Source: CAD feature listing. Evaluate the final solid. Frame: model axes, mm. Round coordinates to 2 decimals unless told otherwise and drop trailing zeros. Order: outer loops, then holes, each group sorted by start corner. A loop starts at its lowest first (then second) coordinate and runs counter-clockwise, first axis right, second up. Notation, with made-up numbers: (22.5, 77) - (60.5, 77) arc R14 ccw to (60.5, 99) - close; hole circle Ø10 at (22, -16.5). An arc over 180 degrees is marked (long way). Return JSON: item names as keys, results as strings. Group by question number.
1) Section D-D, the plane x = 53.5. Return loops of the section in (y, z), plus the area to 3 significant figures.
2) Section A-A, the plane z = -17.5. Return loops of the section in (x, y).
3) Ray query, line 1 (Z direction, x = 0, y = 0.65); line 2 (Z direction, x = -65, y = 1.4); line 3 (X direction, y = 1, z = 19.5). Return the intervals inside material, ascending. Write a range as from..to.
4) Section B-B, the plane x = -65. Return loops of the section in (y, z), plus the area to 3 significant figures.
5) Section C-C, the plane y = 0.9. Give the number of separate pieces and of enclosed holes in the cut face, plus the area to 3 significant figures.
6) Contact query for flat-ended pins moving along their axis: P1, Ø5.5, axis at x = 30.31, z = -17.5, coming from the -Y side; P2, Ø20, axis at x = -65, z = -38, coming from the +Y side; P3, Ø1, axis at x = -58, y = 1.5, coming from the +Z side. Output: stop coordinate, or through.
```python
from build123d import *

# Parameters (mm, degrees)
F1_R     = 6.25
F1_R_2   = 3
F2_DEPTH = 2


with BuildPart() as f2:
    # F1 (on Front) → F2 (new body)
    with BuildSketch(Plane.XZ):
        with BuildLine():
            Line((-60, 67.371839), (-70, 67.371839))
            ThreePointArc((-70, 67.371839), (-77.071068, 64.442907), (-80, 57.371839))
            Line((-80, 57.371839), (-80, 0))
            Line((-80, 0), (-80, -43))
            ThreePointArc((-80, -43), (-77.071068, -50.071068), (-70, -53))
            Line((-70, -53), (0, -53))
            Line((0, -53), (70, -53))
            ThreePointArc((70, -53), (77.071068, -50.071068), (80, -43))
            Line((80, -43), (80, 0))
            Line((80, 0), (80, 57.371839))
            ThreePointArc((80, 57.371839), (77.071068, 64.442907), (70, 67.371839))
            Line((70, 67.371839), (60, 67.371839))
            ThreePointArc((60, 67.371839), (52.928932, 64.442907), (50, 57.371839))
            Line((50, 57.371839), (50, 56.150236))
            ThreePointArc((50, 56.150236), (47.666959, 50.503505), (42.028607, 48.150288))
            Line((42.028607, 48.150288), (0, 48))
            Line((0, 48), (-42.028607, 48.150288))
            ThreePointArc((-42.028607, 48.150288), (-47.666959, 50.503505), (-50, 56.150236))
            Line((-50, 56.150236), (-50, 57.371839))
            ThreePointArc((-50, 57.371839), (-52.928932, 64.442907), (-60, 67.371839))
        make_face()
        with Locations((-65, -38)):
            Circle(F1_R, mode=Mode.SUBTRACT)
        with Locations((-30.310889, -17.5)):
            Circle(F1_R_2, mode=Mode.SUBTRACT)
        with Locations((0, -35)):
            Circle(F1_R_2, mode=Mode.SUBTRACT)
        with Locations((65, -38)):
            Circle(F1_R, mode=Mode.SUBTRACT)
        with Locations((30.310889, -17.5)):
            Circle(F1_R_2, mode=Mode.SUBTRACT)
        with Locations((-30.310889, 17.5)):
            Circle(F1_R_2, mode=Mode.SUBTRACT)
        with Locations((-65, 52.371839)):
            Circle(F1_R, mode=Mode.SUBTRACT)
        with Locations((30.310889, 17.5)):
            Circle(F1_R_2, mode=Mode.SUBTRACT)
        with BuildLine():
            ThreePointArc((3, 35), (-2.12132, 32.87868), (0, 38))
            ThreePointArc((0, 38), (2.12132, 37.12132), (3, 35))
        make_face(mode=Mode.SUBTRACT)
        with Locations((65, 52.371839)):
            Circle(F1_R, mode=Mode.SUBTRACT)
    extrude(amount=-F2_DEPTH)


solid = f2.part
```
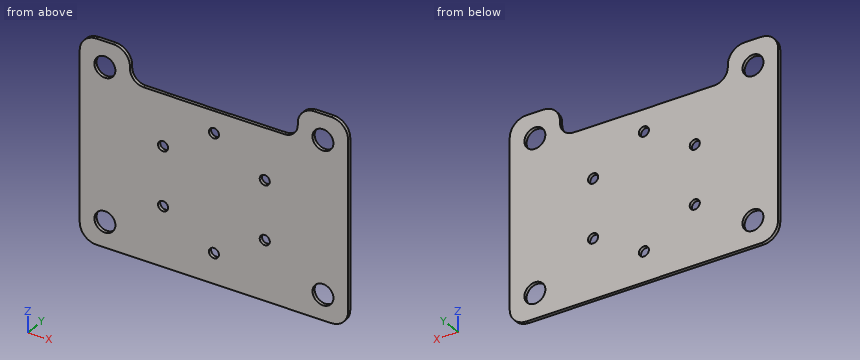
Geometry check:
{
 "1": {"outline": "(0, -53) - (2, -53) - (2, 64.97) - (0, 64.97) - close", "area": "236 mm2"},
 "2": {"outline": "(-80, 0) - (-33.31, 0) - (-33.31, 2) - (-80, 2) - close; (-27.31, 0) - (27.31, 0) - (27.31, 2) - (-27.31, 2) - close; (33.31, 0) - (80, 0) - (80, 2) - (33.31, 2) - close"},
 "3": {"line 1": "-53..-38, -32..32, 38..48", "line 2": "-53..-44.25, -31.75..46.12, 58.62..67.37", "line 3": "-80..-32.55, -28.07..28.07, 32.55..80"},
 "4": {"outline": "(0, -53) - (2, -53) - (2, -44.25) - (0, -44.25) - close; (0, -31.75) - (2, -31.75) - (2, 46.12) - (0, 46.12) - close; (0, 58.62) - (2, 58.62) - (2, 67.37) - (0, 67.37) - close", "area": "191 mm2"},
 "5": {"separate pieces": "1", "enclosed holes": "10", "area": "16,600 mm2"},
 "6": {"P1": "through", "P2": "y = 2", "P3": "z = 67.26"}
}
